Source: CAD feature listing. Evaluate the final solid. Frame: model axes, mm. A direction names the side the tool comes from. Round coordinates to 2 decimals unless told otherwise and drop trailing zeros. Write each loop counter-clockwise with the first axis right and the second up, starting at its lowest first coordinate (ties: lowest second). Pieces come first, ordered by that corner, then holes. Notation, with made-up numbers: M -39.5,82 L -30.5,82 A17 cw -30.5,104 Z; hole C -27.5,29.5 d10. An arc over 180 degrees is marked long. Answer in a Markdown table with one row per item.
from build123d import *

# Parameters (mm, degrees)
SKETCH1_W           = 1524
SKETCH1_H           = 1524
BOSS_EXTRUDE1_DEPTH = 101.6
SKETCH2_W           = 1320.8
SKETCH2_H           = 711.2
CUT_EXTRUDE1_DEPTH  = 2158.65487509
SKETCH3_W           = 101.6
SKETCH3_H           = 101.6
BOSS_EXTRUDE2_DEPTH = 1524
SKETCH4_W           = 1524
SKETCH4_H           = 101.6
BOSS_EXTRUDE3_DEPTH = 50.8


with BuildPart() as part:
    # Sketch1 → Boss-Extrude1 (new body)
    with BuildSketch(Plane.XY):
        with Locations((762, 762)):
            Rectangle(SKETCH1_W, SKETCH1_H)
    extrude(amount=BOSS_EXTRUDE1_DEPTH)

    # Sketch2 → Cut-Extrude1 (cut, through all)
    with BuildSketch(Plane.XY.offset(101.6)):
        with Locations((762, 1168.4)):
            Rectangle(SKETCH2_W, SKETCH2_H)
        with Locations((762, 355.6)):
            Rectangle(SKETCH2_W, SKETCH2_H)
    extrude(amount=-CUT_EXTRUDE1_DEPTH, mode=Mode.SUBTRACT)

    # Sketch3 → Boss-Extrude2 (add)
    with BuildSketch(Plane.XY.offset(101.6)):
        with Locations((50.8, 762)):
            Rectangle(SKETCH3_W, SKETCH3_H)
        with Locations((1473.2, 762)):
            Rectangle(SKETCH3_W, SKETCH3_H)
    extrude(amount=BOSS_EXTRUDE2_DEPTH)

    # Sketch4 → Boss-Extrude3 (add)
    with BuildSketch(Plane.XY.offset(1625.6)):
        with Locations((762, 762)):
            Rectangle(SKETCH4_W, SKETCH4_H)
    extrude(amount=BOSS_EXTRUDE3_DEPTH)

    # Sketch6 → Loft1 section 0
    with BuildSketch(Plane(origin=(0, 812.8, 0), x_dir=(1, 0, 0), z_dir=(0, 1, 0))):
        with BuildLine():
            Line((1524, -1676.4), (1422.4, -1676.4))
            Line((1422.4, -1676.4), (1422.4, -1574.8))
            Line((1422.4, -1574.8), (1524, -1574.8))
            Line((1524, -1574.8), (1524, -1676.4))
        make_face()
    # Sketch5 → Loft1 section 1
    with BuildSketch(Plane.XY.offset(101.6)):
        with BuildLine():
            Line((1422.4, 1524), (1524, 1524))
            Line((1524, 1524), (1524, 1422.4))
            Line((1524, 1422.4), (1422.4, 1422.4))
            Line((1422.4, 1422.4), (1422.4, 1524))
        make_face()
    loft()

    # Sketch14 → Loft2 section 0
    with BuildSketch(Plane(origin=(0, 812.8, 0), x_dir=(1, 0, 0), z_dir=(0, 1, 0))):
        with BuildLine():
            Line((0, -1676.4), (101.6, -1676.4))
            Line((101.6, -1676.4), (101.6, -1574.8))
            Line((101.6, -1574.8), (0, -1574.8))
            Line((0, -1574.8), (0, -1676.4))
        make_face()
    # Sketch13 → Loft2 section 1
    with BuildSketch(Plane.XY.offset(101.6)):
        with BuildLine():
            Line((0, 1524), (101.6, 1524))
            Line((101.6, 1524), (101.6, 1422.4))
            Line((101.6, 1422.4), (0, 1422.4))
            Line((0, 1422.4), (0, 1524))
        make_face()
    loft()


solid = part.part
Q1. Section D-D (y = 1214.5). Return loops of the section in (x, z) (3 decimals).
Solutions:
| item | result |
|---|---|
| outline | M 0,0 L 101.6,0 L 101.6,101.6 L 0,101.6 Z; M 0,604.025 L 101.6,604.025 L 101.6,786.921 L 0,786.921 Z; M 1422.4,0 L 1524,0 L 1524,101.6 L 1422.4,101.6 Z; M 1422.4,604.025 L 1524,604.025 L 1524,786.921 L 1422.4,786.921 Z |
Q2. Material intervals for probe 1 along Y at (x, z) = (496, 95); probe 2 along X at (y, z) = (976, 1237); probe 3 along Y at (x, z) = (96.5, 799), sorted ascending.
Solutions:
| item | result |
|---|---|
| probe 1 | y = 711.2 to 812.8 |
| probe 2 | x = 0 to 101.6, 1422.4 to 1524 |
| probe 3 | y = 711.2 to 812.8, 1133.82 to 1209.05 |
Q3. Access query for faces 4 (the flat face through (1472, 1122, 101.6)), 5 (the flat face through (101.6, 811, 605)), 6 (the flat face through (753, 812.8, 1651)), 7 (the flat face through (1422.4, 351, 52)), 8 (the flat face through (758, 711.2, 1644)). Directions: +Z, -Z, +X, -X, +Y, -Y. A direction counts if a zero-diameter tool reaches every point of the face in a straight line with its end or side. Return the directions, or none.
Solutions:
| item | result |
|---|---|
| face 4 | +X, -X |
| face 5 | +Y |
| face 6 | +Z, -Z, +Y |
| face 7 | +Z, -Z, -Y |
| face 8 | +Z, +X, -X, -Y |
Q4. Section A-A (x = 507.5). Return loops of the section in (y, z).
Solutions:
| item | result |
|---|---|
| outline | M 711.2,0 L 812.8,0 L 812.8,101.6 L 711.2,101.6 Z; M 711.2,1625.6 L 812.8,1625.6 L 812.8,1676.4 L 711.2,1676.4 Z |
Q5. Section B-B (y = 100). Return loops of the section in (x, z).
Solutions:
| item | result |
|---|---|
| outline | M 0,0 L 101.6,0 L 101.6,101.6 L 0,101.6 Z; M 1422.4,0 L 1524,0 L 1524,101.6 L 1422.4,101.6 Z |
Q6. Pull-direction query (Z, two-part tool) for faces 1 (the flat face through (1472, 812.8, 828)), 2 (the flat face through (1472, 361, 101.6)), 3 (the flat face through (101.6, 351, 52)); classes: pulls with the +Z half, pulls with the -Z half, needs draft (parallel to the pull), parting line crosses it, or undercut.
Solutions:
| item | result |
|---|---|
| face 1 | undercut |
| face 2 | pulls with the +Z half |
| face 3 | needs draft |
Q7. Section C-C (z = 1372). Return loops of the section in (x, y), and give its area (3 significant figures).
Solutions:
| item | result |
|---|---|
| outline | M 0,711.2 L 101.6,711.2 L 101.6,812.8 L 0,812.8 Z; M 0,896.72 L 101.6,896.72 L 101.6,950.27 L 0,950.27 Z; M 1422.4,711.2 L 1524,711.2 L 1524,812.8 L 1422.4,812.8 Z; M 1422.4,896.72 L 1524,896.72 L 1524,950.27 L 1422.4,950.27 Z |
| area | 31,500 mm2 |
